Build history of the part. All positions in model axes, mm. Give positions to 0.01 mm unless a question says otherwise; leave off trailing zeros. Write each loop counter-clockwise with the first axis right and the second up, starting at its lowest first coordinate (ties: lowest second). Pieces come first, ordered by that corner, then holes.
from build123d import *

# Parameters (mm, degrees)
F2_W    = 2.5
F2_H    = 30
F4_SIZE = 1
F5_R    = 1


with BuildPart() as f1:
    # F0 (on Front) → F1 (revolve)
    with BuildSketch(Plane.XZ):
        with BuildLine():
            Line((0, 12.7), (0, -12.7))
            ThreePointArc((0, -12.7), (12.7, 0), (0, 12.7))
        make_face()
    revolve(axis=Axis((0, 0, 15.411814), (0, 0, 1)))

    # F2 (on Front) → F3 (revolve)
    with BuildSketch(Plane.XZ):
        with Locations((-3.75, 15)):
            Rectangle(F2_W, F2_H)
    revolve(axis=Axis((0, 0, 22.430043), (0, 0, 1)))

    # F4
    f4_edges = [f1.edges().sort_by_distance(p)[0] for p in [
        (5, 0, 30),
    ]]
    chamfer(f4_edges, length=F4_SIZE)

    # F5
    f5_edges = [f1.edges().sort_by_distance(p)[0] for p in [
        (0, 5, 11.674331),
        (0, -5, 11.674331),
    ]]
    fillet(f5_edges, radius=F5_R)


solid = f1.part
(1) Saw through at B-B, the plane x = -6.75. List the corners of the cut face in (y, z), plus the area to 3 significant figures.
(2) Mould opens along Y. For faces 1 (the face through (0.54, 2.44, 21.35)), 2 (the face through (-2, -2, 30)), 3 (the face through (1.08, 4.88, 20.77)) say: +Y half, -Y half, draft (parallel to the pull), parting line (faces both ways), or undercut.
(3) Saw through at A-A, the plane z = 20.5. List the corners of the cut face in (x, y).
(4) Drop flat-ended pins along their axis: pin 1 (6 mm diameter, centred on y = -3.5, z = -3, fed in from +X); pin 2 (6 mm diameter, centred on x = -7.5, z = 16.5, fed in from +Y); pin 3 (3 mm diameter, centred on x = 5, z = 1.5, fed in from +Y); pin 4 (2 mm diameter, centred on x = 7.5, z = 22, fed in from -Y). Give the stop position or say it passes through.
(5) Probe line 1 (X direction, y = 0, z = 21.25); line 2 (X direction, y = -1, z = 14.5). List the from-to ranges inside material, lowest first.
(6) Saw through at C-C, the plane y = 6.5. List the corners of the cut face in (x, z), plus the area to 3 significant figures.
Computed values:
1. outline: circle Ø21.52 at (0, 0)
1. area: 364 mm2
2. face 1: undercut
2. face 2: draft
2. face 3: parting line
3. outline: circle Ø10 at (0, 0); hole circle Ø5 at (0, 0)
4. pin 1: stops at x = 12.6
4. pin 2: stops at y = 2.18
4. pin 3: stops at y = 12.14
4. pin 4: passes through
5. line 1: x = -5 to -2.5, 2.5 to 5
5. line 2: x = -4.9 to -2.29, 2.29 to 4.9
6. outline: circle Ø21.82 at (0, 0)
6. area: 374 mm2
